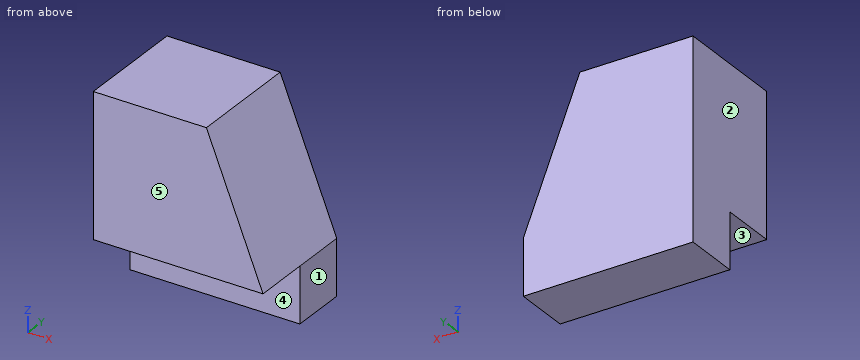
```python
from build123d import *

# Parameters (mm, degrees)
F0_W     = 38.1
F0_H     = 44.45
F1_DEPTH = 12.7
F3_DEPTH = 25.4
F5_DEPTH = 12.7


with BuildPart() as f1:
    # F0 (on Front) → F1 (new body)
    with BuildSketch(Plane.XZ):
        with Locations((19.05, 22.225)):
            Rectangle(F0_W, F0_H)
    extrude(amount=F1_DEPTH)

    # F2 (on face) → F3 (cut)
    with BuildSketch(Plane.XZ.offset(12.7)):
        Polygon((38.1, 44.45), (25.4, 44.45), (38.1, 12.495001), align=None)
    extrude(amount=-F3_DEPTH, mode=Mode.SUBTRACT)

    # F4 (on face) → F5 (join)
    with BuildSketch(Plane.XZ.offset(12.7)):
        Polygon((0, 12.495001), (38.1, 12.495001), (25.4, 44.45), (0, 44.45), align=None)
    extrude(amount=F5_DEPTH)


solid = f1.part
```
Read the model definition and answer for the solid it produces. Units are mm, in the model's axes. Face numbers are marked on the shaded views. A direction names the side the tool comes from. Coordinates: 2 decimals unless noted, no trailing zeros. Order: outer loops, then holes, each group sorted by start corner. A loop starts at its lowest first (then second) coordinate and runs counter-clockwise, first axis right, second up. Notation, with made-up numbers: (89.25, 21) - (95.25, 21) arc R18 ccw to (95.25, 25) - close; hole circle Ø8 at (-22.75, 67.25). An arc over 180 degrees is marked (long way). Answer as a JSON object with one key per item and string values. Group by question number.
Item 1: Flat-ended cylindrical pins translate along their axes: P1, Ø1.5, axis at x = 26.5, z = 16.5, coming from the +Y side; P2, Ø1, axis at x = 6, z = 6.5, coming from the -Y side; P3, Ø5, axis at y = -6, z = 23, coming from the +X side. Find the tip coordinate at first contact, or state that the pin passes through.
Item 2: Consider probe 1 along Z at (x, y) = (3, -18.5) (3 decimals); probe 2 along Y at (x, z) = (4, 4); probe 3 along X at (y, z) = (-23.25, 20). Determine where each line is inside the solid, lowest interval first. Write a range as from..to.
Item 3: The mould has two halves that part along X. Classify the marked faces 1, 2 and 3: +X half, -X half, draft (parallel to the pull), parting line (faces both ways), or undercut.
Item 4: Section A-A (y = -9.75) is taken. Give the vertices of the cut face in (x, z) (3 decimals), plus the area to 3 significant figures.
Item 5: Section D-D (y = -21.5) is taken. Give the vertices of the cut face in (x, z) (3 decimals), plus the area to 3 significant figures.
Item 6: A tool of negligible diameter and unlimited length cuts with its end or side. For the marked faces 4 and 5, from which of +Z, -Z, +X, -X, +Y, -Y can it reach the whole face along a straight path? Write none if from no direction.
Item 7: Section B-B (x = 24.5) is taken. Give the vertices of the cut face in (y, z) (3 decimals), plus the area to 3 significant figures.
Item 8: Section C-C (z = 11.5) is taken. Give the vertices of the cut face in (x, y).
Results are:
{
 "1": {"P1": "stops at y = 0", "P2": "stops at y = -12.7", "P3": "stops at x = 34.92"},
 "2": {"probe 1": "z = 12.495..44.45", "probe 2": "y = -12.7..0", "probe 3": "x = 0..35.12"},
 "3": {"face 1": "+X half", "face 2": "-X half", "face 3": "draft"},
 "4": {"outline": "(0, 0) - (38.1, 0) - (38.1, 12.495) - (25.4, 44.45) - (0, 44.45) - close", "area": "1,490 mm^2"},
 "5": {"outline": "(0, 12.495) - (38.1, 12.495) - (25.4, 44.45) - (0, 44.45) - close", "area": "1,010 mm^2"},
 "6": {"face 4": "-Z, +X, -X, -Y", "face 5": "+Z, -Z, +X, -X, -Y"},
 "7": {"outline": "(-25.4, 12.495) - (-12.7, 12.495) - (-12.7, 0) - (0, 0) - (0, 44.45) - (-25.4, 44.45) - close", "area": "970 mm^2"},
 "8": {"outline": "(0, -12.7) - (38.1, -12.7) - (38.1, 0) - (0, 0) - close"}
}
